Check sheet for the drawn part. Datum: minimum x, y, z corner. Units: mm. Round coordinates to 2 decimals unless told otherwise and drop trailing zeros. Write each loop counter-clockwise with the first axis right and the second up, starting at its lowest first coordinate (ties: lowest second). Pieces come first, ordered by that corner, then holes. Notation, with made-up numbers: (-36.75, 37.25) - (-10.75, 37.25) arc R21 ccw to (-10.75, 42.25) - close; hole circle Ø2 at (41, 42). An arc over 180 degrees is marked (long way). Answer as a JSON object with one key per item and string values. Group by question number.
1) Section check C-C (y = 14.25). Enter the section's corners in (x, z).
2) Section check A-A (z = 3). Enter the section's corners in (x, y).
3) Section check B-B (x = 3). Enter the section's corners in (y, z).
4) Go/stop test with a flat-tipped pin: pin 1 Ø2 at (y, z) = (25.5, 1) entering from -X. Record where the tip stops, or that it passes through.
5) Thickness scan on line 1 (Y direction, x = 5.3, z = 3.7); line 2 (Y direction, x = 0.75, z = 4.45); line 3 (X direction, y = 28.75, z = 2.6). Record the ranges inside material, lowest first.
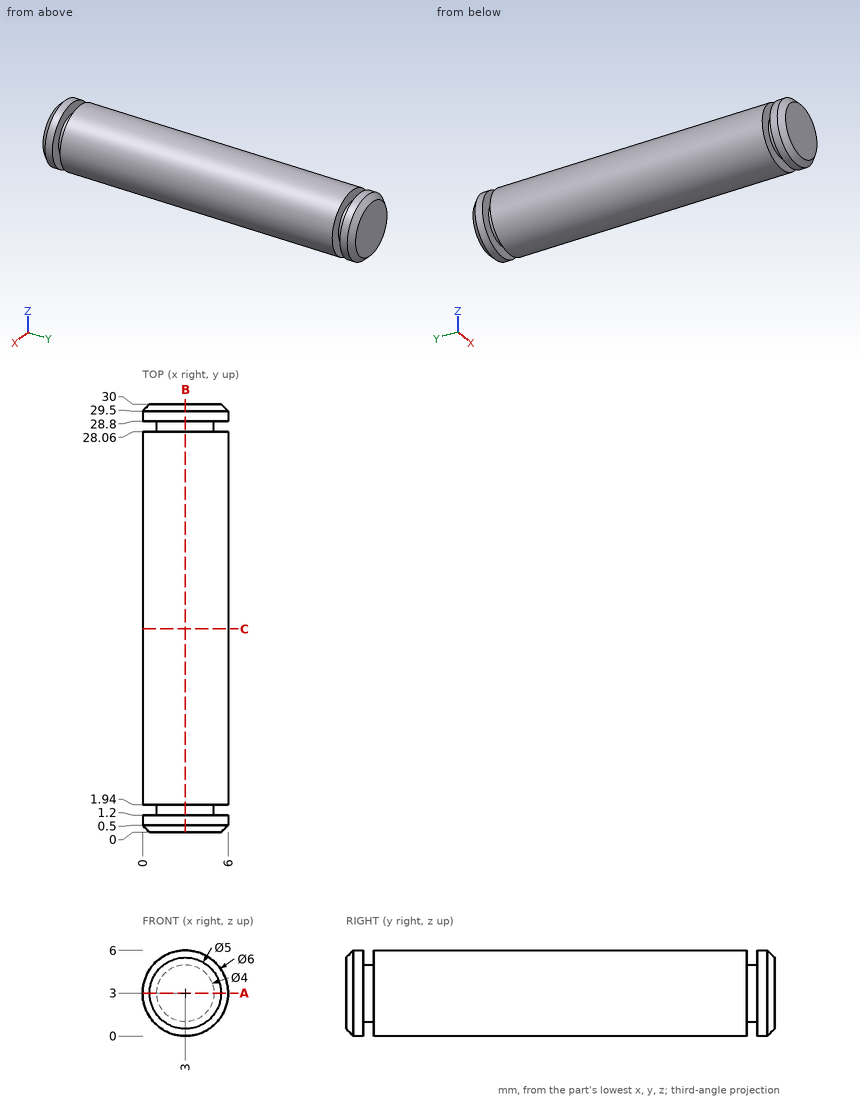
Returned:
{
 "1": {"outline": "circle Ø6 at (3, 3)"},
 "2": {"outline": "(0, 0.5) - (0.5, 0) - (5.5, 0) - (6, 0.5) - (6, 1.2) - (5, 1.2) - (5, 1.94) - (6, 1.94) - (6, 28.06) - (5, 28.06) - (5, 28.8) - (6, 28.8) - (6, 29.5) - (5.5, 30) - (0.5, 30) - (0, 29.5) - (0, 28.8) - (1, 28.8) - (1, 28.06) - (0, 28.06) - (0, 1.94) - (1, 1.94) - (1, 1.2) - (0, 1.2) - close"},
 "3": {"outline": "(0, 0.5) - (0.5, 0) - (1.2, 0) - (1.2, 1) - (1.94, 1) - (1.94, 0) - (28.06, 0) - (28.06, 1) - (28.8, 1) - (28.8, 0) - (29.5, 0) - (30, 0.5) - (30, 5.5) - (29.5, 6) - (28.8, 6) - (28.8, 5) - (28.06, 5) - (28.06, 6) - (1.94, 6) - (1.94, 5) - (1.2, 5) - (1.2, 6) - (0.5, 6) - (0, 5.5) - close"},
 "4": {"pin 1": "x = 0.17"},
 "5": {"line 1": "0 to 1.2, 1.94 to 28.06, 28.8 to 30", "line 2": "0.18 to 1.2, 1.94 to 28.06, 28.8 to 29.82", "line 3": "1.04 to 4.96"}
}
